```python
from build123d import *

# Parameters (mm, degrees)
SKETCH1_W                = 60
SKETCH1_H                = 34
BOSS_EXTRUDE1_DEPTH      = 3
CUT_EXTRUDE1_REACH       = 5
M2_CLEARANCE_HOLE1_D     = 2.2
M2_CLEARANCE_HOLE1_DEPTH = 3
M3_CLEARANCE_HOLE1_D     = 3.2
M3_CLEARANCE_HOLE1_DEPTH = 3
CUT_EXTRUDE2_DEPTH       = 0.2
FILLET2_R                = 4


with BuildPart() as part:
    # Sketch1 → Boss-Extrude1 (new body)
    with BuildSketch(Plane.XY):
        Rectangle(SKETCH1_W, SKETCH1_H)
    extrude(amount=BOSS_EXTRUDE1_DEPTH)

    # Sketch2 → Cut-Extrude1 (cut, up to next)
    with BuildSketch(Plane.XY.offset(3), mode=Mode.PRIVATE) as cut_extrude1_sk1:
        with BuildLine():
            Line((21, 17), (22.5, 15.5))
            Line((22.5, 15.5), (22.5, 12))
            ThreePointArc((22.5, 12), (23.232233047, 10.232233047), (25, 9.5))
            Line((25, 9.5), (28.5, 9.5))
            Line((28.5, 9.5), (30, 8))
            Line((30, 8), (30, 17))
            Line((30, 17), (21, 17))
        make_face()
    cut_extrude1_tool1 = extrude(cut_extrude1_sk1.sketch, amount=-CUT_EXTRUDE1_REACH, mode=Mode.PRIVATE) & part.part
    add(cut_extrude1_tool1.solids().sort_by_distance((26.30521, 13.30521, 3))[0], mode=Mode.SUBTRACT)
    # Sketch2 → Cut-Extrude1 (cut, up to next)
    with BuildSketch(Plane.XY.offset(3), mode=Mode.PRIVATE) as cut_extrude1_sk2:
        with BuildLine():
            Line((-30, 17), (-21, 17))
            Line((-21, 17), (-22.5, 15.5))
            Line((-22.5, 15.5), (-22.5, 12))
            ThreePointArc((-22.5, 12), (-23.232233047, 10.232233047), (-25, 9.5))
            Line((-25, 9.5), (-28.5, 9.5))
            Line((-28.5, 9.5), (-30, 8))
            Line((-30, 8), (-30, 17))
        make_face()
    cut_extrude1_tool2 = extrude(cut_extrude1_sk2.sketch, amount=-CUT_EXTRUDE1_REACH, mode=Mode.PRIVATE) & part.part
    add(cut_extrude1_tool2.solids().sort_by_distance((-26.30521, 13.30521, 3))[0], mode=Mode.SUBTRACT)
    # Sketch2 → Cut-Extrude1 (cut, up to next)
    with BuildSketch(Plane.XY.offset(3), mode=Mode.PRIVATE) as cut_extrude1_sk3:
        with BuildLine():
            Line((30, -8), (30, -17))
            Line((30, -17), (21, -17))
            Line((21, -17), (22.5, -15.5))
            Line((22.5, -15.5), (22.5, -12))
            ThreePointArc((22.5, -12), (23.232233047, -10.232233047), (25, -9.5))
            Line((25, -9.5), (28.5, -9.5))
            Line((28.5, -9.5), (30, -8))
        make_face()
    cut_extrude1_tool3 = extrude(cut_extrude1_sk3.sketch, amount=-CUT_EXTRUDE1_REACH, mode=Mode.PRIVATE) & part.part
    add(cut_extrude1_tool3.solids().sort_by_distance((26.30521, -13.30521, 3))[0], mode=Mode.SUBTRACT)
    # Sketch2 → Cut-Extrude1 (cut, up to next)
    with BuildSketch(Plane.XY.offset(3), mode=Mode.PRIVATE) as cut_extrude1_sk4:
        with BuildLine():
            Line((-22.5, -15.5), (-22.5, -12))
            ThreePointArc((-22.5, -12), (-23.232233047, -10.232233047), (-25, -9.5))
            Line((-25, -9.5), (-28.5, -9.5))
            Line((-28.5, -9.5), (-30, -8))
            Line((-30, -8), (-30, -17))
            Line((-30, -17), (-21, -17))
            Line((-21, -17), (-22.5, -15.5))
        make_face()
    cut_extrude1_tool4 = extrude(cut_extrude1_sk4.sketch, amount=-CUT_EXTRUDE1_REACH, mode=Mode.PRIVATE) & part.part
    add(cut_extrude1_tool4.solids().sort_by_distance((-26.30521, -13.30521, 3))[0], mode=Mode.SUBTRACT)

    # M2 Clearance Hole1
    with Locations(Plane.XY.offset(3)):
        with Locations((19, 13.5), (-19, -13.5), (-19, 13.5), (19, -13.5)):
            Hole(M2_CLEARANCE_HOLE1_D / 2, depth=M2_CLEARANCE_HOLE1_DEPTH)

    # M3 Clearance Hole1
    with Locations(Plane.XY.offset(3)):
        with Locations((-27.5, 0), (27.5, 0)):
            Hole(M3_CLEARANCE_HOLE1_D / 2, depth=M3_CLEARANCE_HOLE1_DEPTH)

    # Sketch7 → Cut-Extrude2 (cut)
    with BuildSketch(Plane(origin=(0, 0, 0), x_dir=(-1, 0, 0), z_dir=(0, 0, -1))):
        with BuildLine():
            Line((-7.5, -13), (7.5, -13))
            ThreePointArc((7.5, -13), (17.577822185, -10.323688824), (25, -3))
            Line((25, -3), (25, 3))
            ThreePointArc((25, 3), (17.577822185, 10.323688824), (7.5, 13))
            Line((7.5, 13), (-7.5, 13))
            ThreePointArc((-7.5, 13), (-17.577822185, 10.323688824), (-25, 3))
            Line((-25, 3), (-25, -3))
            ThreePointArc((-25, -3), (-17.577822185, -10.323688824), (-7.5, -13))
        make_face()
    extrude(amount=-CUT_EXTRUDE2_DEPTH, mode=Mode.SUBTRACT)

    # Fillet2
    fillet2_edges = [part.edges().sort_by_distance(p)[0] for p in [
        (25, -3, 0.1),
        (25, 3, 0.1),
        (-25, 3, 0.1),
        (-25, -3, 0.1),
    ]]
    fillet(fillet2_edges, radius=FILLET2_R)


solid = part.part
```
Build history of the part. All positions in model axes, mm. A direction names the side the tool comes from. Give positions to 0.01 mm unless a question says otherwise; leave off trailing zeros. Order: outer loops, then holes, each group sorted by start corner. A loop starts at its lowest first (then second) coordinate and runs counter-clockwise, first axis right, second up. Notation, with made-up numbers: M -8.5,59.5 L 14.5,59.5 A8 ccw 14.5,67.5 Z; hole C 50.5,68.5 d6. An arc over 180 degrees is marked long. Return JSON: item names as keys, results as strings.
Q1. Two-plate mould, pull along X, no slides. Class faces 3 (the face through (27, -9.5, 2)), 4 (the face through (-22.5, 14, 2)), 5 (the face through (-18.13, 12.83, 1.48)): pulls with the +X half, pulls with the -X half, needs draft (parallel to the pull), parting line crosses it, or undercut.
Answer list:
{"face 3": "needs draft", "face 4": "pulls with the -X half", "face 5": "undercut"}
Q2. Wall check: probe 1 along Y at (x, z) = (19, 1.6); probe 2 along Y at (x, z) = (27.5, 1.9); probe 3 along X at (y, z) = (12.5, 1.9). Give the ranges that are in metal, low to high. Write a range as from..to.
Answer list:
{"probe 1": "y = -17..-14.6, -12.4..12.4, 14.6..17", "probe 2": "y = -9.5..-1.6, 1.6..9.5", "probe 3": "x = -22.5..-19.46, -18.54..18.54, 19.46..22.5"}
Q3. Band-saw the part on B-B (x = -27.5). Give the cut face in (y, z).
Answer list:
{"outline": "M -9.5,0 L -1.6,0 L -1.6,3 L -9.5,3 Z; M 1.6,0 L 9.5,0 L 9.5,3 L 1.6,3 Z"}
Q4. Flat gauge pins, fed straight in: pin 1 (2 mm diameter, centred on x = 19, y = 13.5, fed in from -Z); pin 2 (1.5 mm diameter, centred on y = 13.5, z = 1, fed in from -X); pin 3 (0.9 mm diameter, centred on x = 26, z = 2, fed in from +Y); pin 4 (13 mm diameter, centred on x = 2, y = 3.5, fed in from -Z). Where does each tip first touch, or does it go through?
Answer list:
{"pin 1": "passes through", "pin 2": "stops at x = -22.5", "pin 3": "stops at y = 9.5", "pin 4": "stops at z = 0.2"}
Q5. Band-saw the part on A-A (y = 0). Give the cut face in (x, z).
Answer list:
{"outline": "M -30,0 L -29.1,0 L -29.1,3 L -30,3 Z; M -25.9,0 L -25,0 L -25,0.2 L 25,0.2 L 25,0 L 25.9,0 L 25.9,3 L -25.9,3 Z; M 29.1,0 L 30,0 L 30,3 L 29.1,3 Z"}
Q6. Band-saw the part on D-D (x = 6). Give the cut face in (y, z), then the cut area to 3 significant figures.
Answer list:
{"outline": "M -17,0 L -13,0 L -13,0.2 L 13,0.2 L 13,0 L 17,0 L 17,3 L -17,3 Z", "area": "96.8 mm^2"}
Q7. 3-axis set-ups, long thin cutter, end or side, ignore diameter. For faces 1 (the face through (0, -17, 1)), 2 (the face through (0, 0, 0.2)): which of +Z, -Z, +X, -X, +Y, -Y reach the whole face in a straight line?
Answer list:
{"face 1": "+Z, -Z, +X, -X, -Y", "face 2": "-Z"}
Q8. Band-saw the part on C-C (z = 2.1). Count the separate pieces of the cut face and the enclosed holes in it, then the cut area to 3 significant figures.
Answer list:
{"separate pieces": "1", "enclosed holes": "6", "area": "1,780 mm^2"}
